```python
from build123d import *

# Parameters (mm, degrees)
STAGE1EX_DEPTH      = 30
STAGE1EX_DRAFT      = -30
STAGE1IN_DEPTH      = 27
STAGE1IN_DRAFT      = -30
STAGE2EX_DEPTH      = 15
STAGE2EX_DRAFT      = -60
STAGE2IN_DEPTH      = 20
STAGE2IN_DRAFT      = -60
SKETCH11_R          = 125
BOSS_EXTRUDE6_DEPTH = 3


with BuildPart() as part:
    # Sketch4 → Stage1Ex (with draft: the straight prism first)
    with BuildSketch(Plane(origin=(0, 0, 0), x_dir=(1, 0, 0), z_dir=(0, 1, 0))):
        Polygon((30.901699437, -95.10565163), (80.901699437, -58.778525229), (100, 0), (80.901699437, 58.778525229), (30.901699437, 95.10565163), (-30.901699437, 95.10565163), (-80.901699437, 58.778525229), (-100, 0), (-80.901699437, -58.778525229), (-30.901699437, -95.10565163), align=None)
    extrude(amount=STAGE1EX_DEPTH)
    # Stage1Ex: the draft: its side faces are tilted about the plane it starts from
    stage1ex_sides = [part.faces().sort_by_distance(p)[0] for p in [
        (55.901699437, 15, 76.942088429),
        (90.450849719, 15, 29.389262615),
        (90.450849719, 15, -29.389262615),
        (55.901699437, 15, -76.942088429),
        (0, 15, -95.10565163),
        (-55.901699437, 15, -76.942088429),
        (-90.450849719, 15, -29.389262615),
        (-90.450849719, 15, 29.389262615),
        (-55.901699437, 15, 76.942088429),
        (0, 15, 95.10565163),
    ]]
    draft(stage1ex_sides, Plane(origin=(0, 0, 0), x_dir=(1, 0, 0), z_dir=(0, 1, 0)), STAGE1EX_DRAFT)


with BuildPart() as stage1in_tool:
    # Sketch7 → Stage1In (with draft: the straight prism first)
    with BuildSketch(Plane(origin=(0, 30, 0), x_dir=(1, 0, 0), z_dir=(0, 1, 0))):
        Polygon((-115.211859946, 0), (-93.20835265, -67.719832166), (-35.602422677, -109.572990156), (35.602422677, -109.572990156), (93.20835265, -67.719832166), (115.211859946, 0), (93.20835265, 67.719832166), (35.602422677, 109.572990156), (-35.602422677, 109.572990156), (-93.20835265, 67.719832166), align=None)
    extrude(amount=-STAGE1IN_DEPTH)
    # Stage1In: the draft: its side faces are tilted about the plane it starts from
    stage1in_sides = [stage1in_tool.faces().sort_by_distance(p)[0] for p in [
        (-104.210106298, 16.5, 33.859916083),
        (-64.405387663, 16.5, 88.646411161),
        (0, 16.5, 109.572990156),
        (64.405387663, 16.5, 88.646411161),
        (104.210106298, 16.5, 33.859916083),
        (104.210106298, 16.5, -33.859916083),
        (64.405387663, 16.5, -88.646411161),
        (0, 16.5, -109.572990156),
        (-64.405387663, 16.5, -88.646411161),
        (-104.210106298, 16.5, -33.859916083),
    ]]
    draft(stage1in_sides, Plane(origin=(0, 30, 0), x_dir=(1, 0, 0), z_dir=(0, 1, 0)), STAGE1IN_DRAFT)


with BuildPart() as part_1:
    add(part.part)

    # Stage1In: cut by stage1in_tool
    add(stage1in_tool.part, mode=Mode.SUBTRACT)


with BuildPart() as stage2ex_tool:
    # Sketch8 → Stage2Ex (with draft: the straight prism first)
    with BuildSketch(Plane(origin=(0, 30, 0), x_dir=(1, 0, 0), z_dir=(0, 1, 0))):
        Polygon((36.52947366, 112.426159705), (-36.52947366, 112.426159705), (-95.635403633, 69.483187922), (-118.211859946, 0), (-95.635403633, -69.483187922), (-36.52947366, -112.426159705), (36.52947366, -112.426159705), (95.635403633, -69.483187922), (118.211859946, 0), (95.635403633, 69.483187922), align=None)
    extrude(amount=STAGE2EX_DEPTH)
    # Stage2Ex: the draft: its side faces are tilted about the plane it starts from
    stage2ex_sides = [stage2ex_tool.faces().sort_by_distance(p)[0] for p in [
        (0, 37.5, -112.426159705),
        (-66.082438647, 37.5, -90.954673814),
        (-106.92363179, 37.5, -34.741593961),
        (-106.92363179, 37.5, 34.741593961),
        (-66.082438647, 37.5, 90.954673814),
        (0, 37.5, 112.426159705),
        (66.082438647, 37.5, 90.954673814),
        (106.92363179, 37.5, 34.741593961),
        (106.92363179, 37.5, -34.741593961),
        (66.082438647, 37.5, -90.954673814),
    ]]
    draft(stage2ex_sides, Plane(origin=(0, 30, 0), x_dir=(1, 0, 0), z_dir=(0, 1, 0)), STAGE2EX_DRAFT)


with BuildPart() as part_2:
    add(part_1.part)

    # Stage2Ex: add stage2ex_tool
    add(stage2ex_tool.part)


with BuildPart() as stage2in_tool:
    # Sketch10 → Stage2In (with draft: the straight prism first)
    with BuildSketch(Plane(origin=(0, 45, 0), x_dir=(1, 0, 0), z_dir=(0, 1, 0))):
        Polygon((115.308908944, -83.776826205), (142.529649866, 0), (115.308908944, 83.776826205), (44.044084011, 135.55375227), (-44.044084011, 135.55375227), (-115.308908944, 83.776826205), (-142.529649866, 0), (-115.308908944, -83.776826205), (-44.044084011, -135.55375227), (44.044084011, -135.55375227), align=None)
    extrude(amount=-STAGE2IN_DEPTH)
    # Stage2In: the draft: its side faces are tilted about the plane it starts from
    stage2in_sides = [stage2in_tool.faces().sort_by_distance(p)[0] for p in [
        (128.919279405, 35, 41.888413103),
        (128.919279405, 35, -41.888413103),
        (79.676496477, 35, -109.665289238),
        (0, 35, -135.55375227),
        (-79.676496477, 35, -109.665289238),
        (-128.919279405, 35, -41.888413103),
        (-128.919279405, 35, 41.888413103),
        (-79.676496477, 35, 109.665289238),
        (0, 35, 135.55375227),
        (79.676496477, 35, 109.665289238),
    ]]
    draft(stage2in_sides, Plane(origin=(0, 45, 0), x_dir=(1, 0, 0), z_dir=(0, 1, 0)), STAGE2IN_DRAFT)


with BuildPart() as part_3:
    add(part_2.part)

    # Stage2In: cut by stage2in_tool
    add(stage2in_tool.part, mode=Mode.SUBTRACT)

    # Sketch11 → Boss-Extrude6 (add)
    with BuildSketch(Plane(origin=(0, 45, 0), x_dir=(1, 0, 0), z_dir=(0, 1, 0))):
        Polygon((117.735959927, -85.540181962), (145.529649866, 0), (117.735959927, 85.540181962), (44.971134994, 138.406921819), (-44.971134994, 138.406921819), (-117.735959927, 85.540181962), (-145.529649866, 0), (-117.735959927, -85.540181962), (-44.971134994, -138.406921819), (44.971134994, -138.406921819), align=None)
        with Locations(Location((0, 0, 0), (0, 0, 270))):
            Circle(SKETCH11_R, mode=Mode.SUBTRACT)
    extrude(amount=BOSS_EXTRUDE6_DEPTH)


solid = part_3.part
```
Build history of the part. All positions in model axes, mm. A direction names the side the tool comes from. Round coordinates to 2 decimals unless told otherwise and drop trailing zeros. Write each loop counter-clockwise with the first axis right and the second up, starting at its lowest first coordinate (ties: lowest second). Pieces come first, ordered by that corner, then holes. Notation, with made-up numbers: (-5, 64) -> (37, 64) arc R22 ccw to (37, 72) -> close; hole circle Ø8 at (69, -27.75). An arc over 180 degrees is marked (long way). Put each result on its own line as item: value.
Item 1: Slice it at A-A, the plane x = 0. Give the cut face in (y, z), plus the area to 3 significant figures.
Here are the results:
outline: (0, -95.11) -> (30, -112.43) -> (45, -138.41) -> (48, -138.41) -> (48, -125) -> (45, -125) -> (45, -135.55) -> (30, -109.57) -> (3, -93.98) -> (3, 93.98) -> (30, 109.57) -> (45, 135.55) -> (45, 125) -> (48, 125) -> (48, 138.41) -> (45, 138.41) -> (30, 112.43) -> (0, 95.11) -> close
area: 896 mm^2
Item 2: Slice it at B-B, the plane y = 11. Give the cut face in (x, z), plus the area to 3 significant figures.
Here are the results:
outline: (-106.68, 0) -> (-86.3, -62.7) -> (-32.97, -101.46) -> (32.97, -101.46) -> (86.3, -62.7) -> (106.68, 0) -> (86.3, 62.7) -> (32.97, 101.46) -> (-32.97, 101.46) -> (-86.3, 62.7) -> close; hole (-103.68, 0) -> (-83.88, -60.94) -> (-32.04, -98.6) -> (32.04, -98.6) -> (83.88, -60.94) -> (103.68, 0) -> (83.88, 60.94) -> (32.04, 98.6) -> (-32.04, 98.6) -> (-83.88, 60.94) -> close
area: 1,850 mm^2
Item 3: Slice it at D-D, the plane y = 36. Give the cut face in (x, z), plus the area to 3 significant figures.
Here are the results:
outline: (-129.14, 0) -> (-104.48, -75.91) -> (-39.91, -122.82) -> (39.91, -122.82) -> (104.48, -75.91) -> (129.14, 0) -> (104.48, 75.91) -> (39.91, 122.82) -> (-39.91, 122.82) -> (-104.48, 75.91) -> close; hole (-126.14, 0) -> (-102.05, -74.14) -> (-38.98, -119.97) -> (38.98, -119.97) -> (102.05, -74.14) -> (126.14, 0) -> (102.05, 74.14) -> (38.98, 119.97) -> (-38.98, 119.97) -> (-102.05, 74.14) -> close
area: 2,250 mm^2
Item 4: Two-plate mould, pull along Z, no slides. Class faces 4 (the face through (-74.12, 37.395, 100.947)), 5 (the face through (0.617, 37.605, -122.745)), 6 (the face through (131.827, 46.479, -42.171)): pulls with the +Z half, pulls with the -Z half, needs draft (parallel to the pull), parting line crosses it, or undercut.
Here are the results:
face 4: pulls with the +Z half
face 5: undercut
face 6: pulls with the -Z half
Item 5: Tool access for faces 1 (the face through (-116.547, 37.605, -38.517)), 2 (the face through (-96.747, 16.689, -31.959)), 3 (the face through (60.51, 14.79, 84.15)): list every direction of +Z, -Z, +X, -X, +Y, -Y with a clear straight run to the whole face (end or side of a thin tool).
Here are the results:
face 1: none
face 2: +Y
face 3: +Z, +X, -Y
Item 6: Flat gauge pins, fed straight in: P1, Ø12, axis at y = 15, z = 47.5, coming from the -X side; P2, Ø1, axis at x = -36, z = 4, coming from the +Y side; P3, Ø4, axis at x = -58.5, y = 36, coming from the +Z side. Where does each tip first touch, or does it go through?
Here are the results:
P1: stops at x = -97.8
P2: stops at y = 3
P3: stops at z = 113.83
Item 7: Slice it at C-C, the plane z = 33. Give the cut face in (x, y).
Here are the results:
outline: (-134.81, 45) -> (-107.49, 30) -> (-89.28, 0) -> (89.28, 0) -> (107.49, 30) -> (134.81, 45) -> (134.81, 48) -> (120.57, 48) -> (120.57, 45) -> (131.81, 45) -> (104.49, 30) -> (88.1, 3) -> (-88.1, 3) -> (-104.49, 30) -> (-131.81, 45) -> (-120.57, 45) -> (-120.57, 48) -> (-134.81, 48) -> close
Item 8: Wall check: probe 1 along X at (y, z) = (46.4, 0); probe 2 along Y at (x, z) = (8, 73.5); probe 3 along Z at (x, y) = (20, 10.5). Give the ranges that are in metal, low to high. Write a range as from..to.
Here are the results:
probe 1: x = -145.53..-125, 125..145.53
probe 2: y = 0..3
probe 3: z = -101.17..-98.31, 98.31..101.17
